Verification items for this drawing (mm, ordinates from the low corner). A direction names the side the tool comes from. Round coordinates to 2 decimals unless told otherwise and drop trailing zeros. Loops run counter-clockwise (first coordinate to the right, second up) from the corner with the lowest first, then second, coordinate; pieces in that order, holes last. Notation, with made-up numbers: (32.5, 45) - (44.5, 45) arc R12 ccw to (44.5, 61) - close; hole circle Ø11 at (52, 59). An arc over 180 degrees is marked (long way). Answer in a Markdown table with one row per item. Add a question column.
(1) Access from +Z, -Z, +X, -X, +Y, -Y to the whole of each face (thin tool, end or side, straight path). Record for the marked faces 1, 2 and 3.
(2) Gauge pin test, flat ends, axial feed: pin 1 (6 mm diameter, centred on x = 85.5, y = 10, fed in from +Z); pin 2 (4 mm diameter, centred on x = 94.5, y = 5.5, fed in from +Z); pin 3 (7 mm diameter, centred on y = 9.5, z = 131.5, fed in from +X). Record the tip position at first contact, or that the pin passes through.
(3) Thickness scan on line 1 along Z through (x, y) = (116, 10.5); line 2 along Z through (x, y) = (83, 7.75). Record the ranges inside material, lowest first.
(4) Cross-section at B-B on x = 98.5. Enter the section's corners in (y, z).
(5) Cross-section at A-A on y = 6.35. Enter the section's corners in (x, z).
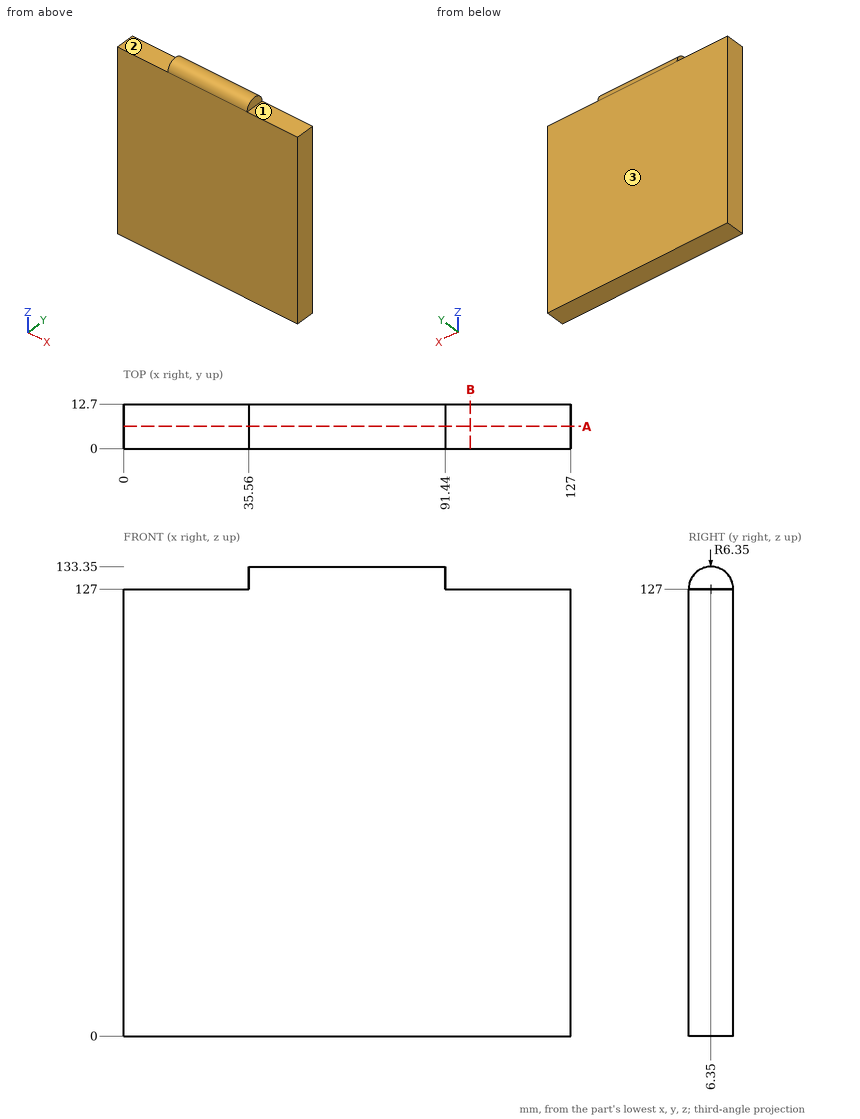
Answers:
| question | item | result |
|---|---|---|
| 1 | face 1 | +Z, +X, +Y, -Y |
| 1 | face 2 | +Z, -X, +Y, -Y |
| 1 | face 3 | +Z, -Z, +X, -X, +Y |
| 2 | pin 1 | stops at z = 133.32 |
| 2 | pin 2 | stops at z = 127 |
| 2 | pin 3 | stops at x = 91.44 |
| 3 | line 1 | z = 0 to 127 |
| 3 | line 2 | z = 0 to 133.19 |
| 4 | outline | (0, 0) - (12.7, 0) - (12.7, 127) - (0, 127) - close |
| 5 | outline | (0, 0) - (127, 0) - (127, 127) - (91.44, 127) - (91.44, 133.35) - (35.56, 133.35) - (35.56, 127) - (0, 127) - close |
